Design review of the part built by this model. Coordinates are the model's own, in mm. A direction names the side the tool comes from. Coordinates: 2 decimals unless noted, no trailing zeros. Write each loop counter-clockwise with the first axis right and the second up, starting at its lowest first coordinate (ties: lowest second). Pieces come first, ordered by that corner, then holes.
Q1. Machinability: for faces 1 (the flat face through (0, 11, 24)), 2 (the flat face through (-8, 5, 24)), 3 (the cylindrical face through (-15.43, 36.78, 14)), which of the approach directions +Z, -Z, +X, -X, +Y, -Y give a long, thin tool a straight path to every point of the face, cutting with its end or side? Answer none if there is none.
Q2. For probe 1 along X at (y, z) = (37.05, 15.5); probe 2 along Z at (x, y) = (-15, 37); probe 3 along Z at (x, y) = (-14.5, 27), list the stretches that pass through material, from the lowest coordinate up.
Q3. Take a section at C-C (x = 9). Give the boundary of the cut face in (y, z), and give its area (3 significant figures).
Q4. Take a section at D-D (y = 45). Give the boundary of the cut face in (x, z), and give its area (3 significant figures).
Q5. Take a section at B-B (z = 0). Give the boundary of the cut face in (x, y).
Q6. Mouldability with a two-part tool opening along Z and no side actions: class faces 4 (the flat face through (8, 5, 24)), 5 (the flat face through (-15, 34.5, 15)), 6 (the flat face through (0, 6, 27.5)) as pulls with the +Z half, pulls with the -Z half, needs draft (parallel to the pull), parting line crosses it, or undercut.
Q7. Insertion check: pin 1 (0.9 mm diameter, centred on x = 15.5, z = -16, fed in from +Y); pin 2 (3.5 mm diameter, centred on x = 15.5, z = 16, fed in from +Y); pin 3 (3 mm diameter, centred on y = 4, z = 25.5, fed in from +X). Each pin has a flat end and moves straight along its axis. Give the tip position at first contact, or say it passes through.
Q8. Take a section at A-A (y = 31.5). Give the boundary of the cut face in (x, z), and give its area (3 significant figures).
```python
from build123d import *

# Parameters (mm, degrees)
BOSS_EXTRUDE1_DEPTH = 39
SKETCH2_R           = 2.5
BOSS_EXTRUDE2_DEPTH = 9
BOSS_EXTRUDE3_DEPTH = 15
SKETCH4_R           = 1.5
CUT_EXTRUDE1_DEPTH  = 4.5
SKETCH5_W           = 16
SKETCH5_H           = 11
BOSS_EXTRUDE4_DEPTH = 6.5


with BuildPart() as part:
    # Sketch1 → Boss-Extrude1 (new body)
    with BuildSketch(Plane(origin=(0, 0, 0), x_dir=(1, 0, 0), z_dir=(0, 1, 0))):
        Polygon((-21, 15.5), (-15.5, 21), (15.5, 21), (21, 15.5), (21, -15.5), (15.5, -21), (-15.5, -21), (-21, -15.5), align=None)
    extrude(amount=BOSS_EXTRUDE1_DEPTH)

    # Sketch2 → Boss-Extrude2 (add)
    with BuildSketch(Plane(origin=(0, 39, 0), x_dir=(1, 0, 0), z_dir=(0, 1, 0))):
        with Locations(Location((0, 0, 0), (0, 0, 90))):
            Circle(SKETCH2_R)
    extrude(amount=BOSS_EXTRUDE2_DEPTH)

    # Sketch3 → Boss-Extrude3 (add)
    with BuildSketch(Plane(origin=(0, 48, 0), x_dir=(1, 0, 0), z_dir=(0, 1, 0))):
        with BuildLine():
            Line((-1.5, 2), (1.5, 2))
            ThreePointArc((1.5, 2), (0, -2.5), (-1.5, 2))
        make_face()
    extrude(amount=BOSS_EXTRUDE3_DEPTH)

    # Sketch4 → Cut-Extrude1 (cut)
    with BuildSketch(Plane(origin=(0, 39, 0), x_dir=(1, 0, 0), z_dir=(0, 1, 0))):
        with Locations(Location((-15.5, 15.5, 0), (0, 0, 270))):
            Circle(SKETCH4_R)
        with Locations(Location((15.5, 15.5, 0), (0, 0, 270))):
            Circle(SKETCH4_R)
        with Locations(Location((15.5, -15.5, 0), (0, 0, 270))):
            Circle(SKETCH4_R)
        with Locations(Location((-15.5, -15.5, 0), (0, 0, 270))):
            Circle(SKETCH4_R)
    extrude(amount=-CUT_EXTRUDE1_DEPTH, mode=Mode.SUBTRACT)

    # Sketch5 → Boss-Extrude4 (add)
    with BuildSketch(Plane.XY.offset(21)):
        with Locations((0, 5.5)):
            Rectangle(SKETCH5_W, SKETCH5_H)
    extrude(amount=BOSS_EXTRUDE4_DEPTH)


solid = part.part
```
Response:
1. face 1: +Z, +X, -X, +Y
1. face 2: +Z, -X, +Y, -Y
1. face 3: +Y
2. probe 1: x = -21 to -17, -14 to 14, 17 to 21
2. probe 2: z = -21 to -16.91, -14.09 to 14.09, 16.91 to 21
2. probe 3: z = -21 to 21
3. outline: (0, -21) - (39, -21) - (39, 21) - (0, 21) - close
3. area: 1,640 mm2
4. outline: circle Ø5 at (0, 0)
4. area: 19.6 mm2
5. outline: (-21, 0) - (21, 0) - (21, 39) - (2.5, 39) - (2.5, 63) - (-2.5, 63) - (-2.5, 39) - (-21, 39) - close
6. face 4: needs draft
6. face 5: undercut
6. face 6: pulls with the +Z half
7. pin 1: stops at y = 34.5
7. pin 2: stops at y = 39
7. pin 3: stops at x = 8
8. outline: (-21, -15.5) - (-15.5, -21) - (15.5, -21) - (21, -15.5) - (21, 15.5) - (15.5, 21) - (-15.5, 21) - (-21, 15.5) - close
8. area: 1,700 mm2
